from build123d import *

# Parameters (mm, degrees)
SKETCH1_R               = 1.5
BOSS_EXTRUDE1_DEPTH     = 3.5
SKETCH2_R               = 7.25
BOSS_EXTRUDE2_DEPTH     = 22.5
SKETCH3_R               = 2.5
CUT_EXTRUDE1_DEPTH      = 27
SKETCH6_R               = 9.569614172
CUT_EXTRUDE6_DEPTH      = 7.5
SKETCH7_R               = 17.775779512
SKETCH7_R_2             = 6.25
CUT_EXTRUDE7_DEPTH      = 7.5
SKETCH8_R               = 1
CUT_EXTRUDE8_DEPTH      = 4.5
SKETCH9_R               = 1.9
CUT_EXTRUDE9_DEPTH      = 13
CUT_EXTRUDE9_DEPTH_BACK = 0.5


with BuildPart() as part:
    # Sketch1 → Boss-Extrude1 (new body)
    with BuildSketch(Plane.XY):
        with BuildLine():
            Line((-14.730127019, -3.5044428), (-4.330127019, 14.508885599))
            ThreePointArc((-4.330127019, 14.508885599), (0, 17.008885599), (4.330127019, 14.508885599))
            Line((4.330127019, 14.508885599), (14.730127019, -3.5044428))
            ThreePointArc((14.730127019, -3.5044428), (14.730127019, -8.5044428), (10.4, -11.0044428))
            Line((10.4, -11.0044428), (-10.4, -11.0044428))
            ThreePointArc((-10.4, -11.0044428), (-14.730127019, -8.5044428), (-14.730127019, -3.5044428))
        make_face()
        with Locations((0, 12.008885599)):
            Circle(SKETCH1_R, mode=Mode.SUBTRACT)
        with Locations((-10.4, -6.0044428)):
            Circle(SKETCH1_R, mode=Mode.SUBTRACT)
        with Locations((10.4, -6.0044428)):
            Circle(SKETCH1_R, mode=Mode.SUBTRACT)
    extrude(amount=BOSS_EXTRUDE1_DEPTH)

    # Sketch2 → Boss-Extrude2 (add)
    with BuildSketch(Plane.XY.offset(3.5)):
        Circle(SKETCH2_R)
    extrude(amount=BOSS_EXTRUDE2_DEPTH)

    # Sketch3 → Cut-Extrude1 (cut, through all)
    with BuildSketch(Plane.XY.offset(26)):
        Circle(SKETCH3_R)
    extrude(amount=-CUT_EXTRUDE1_DEPTH, mode=Mode.SUBTRACT)

    # Sketch6 → Cut-Extrude6 (cut)
    with BuildSketch(Plane.XY.offset(24)):
        Circle(SKETCH6_R)
        Polygon((7.5, 0), (4.452808103, 0.65), (4.435733208, 0.757806641), (7.132923872, 2.317627458), (4.034011116, 1.994180112), (3.984457842, 2.091433888), (6.067627458, 4.408389392), (3.220337014, 3.14315598), (3.14315598, 3.220337014), (4.408389392, 6.067627458), (2.091433888, 3.984457842), (1.994180112, 4.034011116), (2.317627458, 7.132923872), (0.757806641, 4.435733208), (0.65, 4.452808103), (0, 7.5), (-0.65, 4.452808103), (-0.757806641, 4.435733208), (-2.317627458, 7.132923872), (-1.994180112, 4.034011116), (-2.091433888, 3.984457842), (-4.408389392, 6.067627458), (-3.14315598, 3.220337014), (-3.220337014, 3.14315598), (-6.067627458, 4.408389392), (-3.984457842, 2.091433888), (-4.034011116, 1.994180112), (-7.132923872, 2.317627458), (-4.435733208, 0.757806641), (-4.452808103, 0.65), (-7.5, 0), (-4.452808103, -0.65), (-4.435733208, -0.757806641), (-7.132923872, -2.317627458), (-4.034011116, -1.994180112), (-3.984457842, -2.091433888), (-6.067627458, -4.408389392), (-3.220337014, -3.14315598), (-3.14315598, -3.220337014), (-4.408389392, -6.067627458), (-2.091433888, -3.984457842), (-1.994180112, -4.034011116), (-2.317627458, -7.132923872), (-0.757806641, -4.435733208), (-0.65, -4.452808103), (0, -7.5), (0.65, -4.452808103), (0.757806641, -4.435733208), (2.317627458, -7.132923872), (1.994180112, -4.034011116), (2.091433888, -3.984457842), (4.408389392, -6.067627458), (3.14315598, -3.220337014), (3.220337014, -3.14315598), (6.067627458, -4.408389392), (3.984457842, -2.091433888), (4.034011116, -1.994180112), (7.132923872, -2.317627458), (4.435733208, -0.757806641), (4.452808103, -0.65), align=None, mode=Mode.SUBTRACT)
    extrude(amount=-CUT_EXTRUDE6_DEPTH, mode=Mode.SUBTRACT)

    # Sketch7 → Cut-Extrude7 (cut)
    with BuildSketch(Plane.XY.offset(24)):
        Circle(SKETCH7_R)
        Circle(SKETCH7_R_2, mode=Mode.SUBTRACT)
    extrude(amount=-CUT_EXTRUDE7_DEPTH, mode=Mode.SUBTRACT)

    # Sketch8 → Cut-Extrude8 (cut, through all)
    with BuildSketch(Plane.XY.offset(3.5)):
        with Locations((7.904405598, 4.5636107)):
            Circle(SKETCH8_R)
        with Locations((0, -9.1272214)):
            Circle(SKETCH8_R)
        with Locations((-7.904405598, 4.5636107)):
            Circle(SKETCH8_R)
    extrude(amount=-CUT_EXTRUDE8_DEPTH, mode=Mode.SUBTRACT)

    # Sketch9 → Cut-Extrude9 (cut, two sides)
    with BuildSketch(Plane.XY.offset(3.5)) as cut_extrude9_sk:
        with Locations((7.904405598, 4.5636107)):
            Circle(SKETCH9_R)
        with Locations((0, -9.1272214)):
            Circle(SKETCH9_R)
        with Locations((-7.904405598, 4.5636107)):
            Circle(SKETCH9_R)
    extrude(amount=CUT_EXTRUDE9_DEPTH, mode=Mode.SUBTRACT)
    extrude(cut_extrude9_sk.sketch, amount=-CUT_EXTRUDE9_DEPTH_BACK, mode=Mode.SUBTRACT)


solid = part.part
Read the model definition and answer for the solid it produces. Units are mm, in the model's axes. A direction names the side the tool comes from. Coordinates: 2 decimals unless noted, no trailing zeros. Write each loop counter-clockwise with the first axis right and the second up, starting at its lowest first coordinate (ties: lowest second). Pieces come first, ordered by that corner, then holes. Notation, with made-up numbers: M -24,0.5 L 29,0.5 A28 cw 29,26.5 Z; hole C -24.5,39.25 d11. An arc over 180 degrees is marked long. Use a Markdown table: item, result.
Q1. The part is cut by section A-A, the plane z = 9. Write down the section's boundary in (x, y).
Answer block:
| item | result |
|---|---|
| outline | M -6.41,3.4 A7.25 ccw -0.26,-7.25 A1.9 cw 0.26,-7.25 A7.25 ccw 6.41,3.4 A1.9 cw 6.14,3.85 A7.25 ccw -6.14,3.85 A1.9 cw Z; hole C 0,0 d5 |
Q2. Which of the six approach directions +Z, -Z, +X, -X, +Y, -Y give full straight-line access (tool end or side, diameter ignored) to faces 4 (the face through (5.361, 0.456, 20.303)), 5 (the face through (3.35, -6.43, 24.99)), 6 (the face through (-4.05, 3.51, 20.3)), 7 (the face through (9.294, -4.991, 1.726))?
Answer block:
| item | result |
|---|---|
| face 4 | +X |
| face 5 | +Z |
| face 6 | none |
| face 7 | +Z, -Z |
Q3. Determine the mould class of faces 1 (the face through (-3.51, -4.05, 20.3)), 2 (the face through (6.23, -3.71, 9.91)), 3 (the face through (8, -5, 3.5)) for opening direction Z: released by +Z, released by -Z, zero draft, split by the parting line, or undercut.
Answer block:
| item | result |
|---|---|
| face 1 | undercut |
| face 2 | zero draft |
| face 3 | released by +Z |
Q4. Each of these flat-tipped pins is pushed along its axis until it touches: pin 1 Ø1 at (x, z) = (4, 15.5) entering from -Y; pin 2 Ø10.5 at (x, y) = (2.5, 8.5) entering from +Z; pin 3 Ø5 at (y, z) = (-5, 10.5) entering from +X; pin 4 Ø10 at (x, z) = (8, 18.5) entering from -Y. Where does it stop, or does it pass through?
Answer block:
| item | result |
|---|---|
| pin 1 | stops at y = -6.35 |
| pin 2 | stops at z = 26 |
| pin 3 | stops at x = 6.81 |
| pin 4 | stops at y = -6.39 |
Q5. Straight lines are drawn through the part: L1, parallel to Y at x = 0, z = 5; L2, parallel to Z at x = 6.5, y = 3.5; L3, parallel to Y at x = 6.5, z = 4. For each, find the intervals that lie inside material, in ascending order. Write a range as [from, to].
Answer block:
| item | result |
|---|---|
| L1 | y = [-7.23, -2.5], [2.5, 7.25] |
| L2 | z = [0, 3] |
| L3 | y = [-3.21, 3.21] |
